from build123d import *

# Parameters (mm, degrees)
BOSS_EXTRUDE1_DEPTH = 10
FILLET1_R           = 5
CUT_EXTRUDE1_REACH  = 273.931
SKETCH2_R           = 1.5
SKETCH3_R           = 3
CUT_EXTRUDE2_DEPTH  = 2


with BuildPart() as part:
    # Sketch1 → Boss-Extrude1 (new body)
    with BuildSketch(Plane.XY):
        with BuildLine():
            Line((20, 35.715152736), (170, 35.715152736))
            ThreePointArc((170, 35.715152736), (184.142135624, 29.85728836), (190, 15.715152736))
            Line((190, 15.715152736), (190, -189.284847264))
            ThreePointArc((190, -189.284847264), (188.535533906, -192.82038117), (185, -194.284847264))
            Line((185, -194.284847264), (5, -194.284847264))
            ThreePointArc((5, -194.284847264), (1.464466094, -192.82038117), (0, -189.284847264))
            Line((0, -189.284847264), (0, 15.715152736))
            ThreePointArc((0, 15.715152736), (5.857864376, 29.85728836), (20, 35.715152736))
        make_face()
    extrude(amount=BOSS_EXTRUDE1_DEPTH)

    # Fillet1
    fillet1_edges = [part.edges().sort_by_distance(p)[0] for p in [
        (1.464466094, -192.82038117, 10),
        (95, -194.284847264, 10),
        (188.535533906, -192.82038117, 10),
        (190, -86.784847264, 10),
        (184.142135624, 29.85728836, 10),
        (95, 35.715152736, 10),
        (5.857864376, 29.85728836, 10),
        (0, -86.784847264, 10),
    ]]
    fillet(fillet1_edges, radius=FILLET1_R)

    # Sketch2 → Cut-Extrude1 (cut, up to next)
    with BuildSketch(Plane.XY.offset(10), mode=Mode.PRIVATE) as cut_extrude1_sk1:
        with Locations((20, -174.284847264)):
            Circle(SKETCH2_R)
    cut_extrude1_tool1 = extrude(cut_extrude1_sk1.sketch, amount=-CUT_EXTRUDE1_REACH, mode=Mode.PRIVATE) & part.part
    # Sketch2 → Cut-Extrude1 (cut, up to next)
    with BuildSketch(Plane.XY.offset(10), mode=Mode.PRIVATE) as cut_extrude1_sk2:
        with Locations((170, -174.284847264)):
            Circle(SKETCH2_R)
    cut_extrude1_tool2 = extrude(cut_extrude1_sk2.sketch, amount=-CUT_EXTRUDE1_REACH, mode=Mode.PRIVATE) & part.part
    # Sketch2 → Cut-Extrude1 (cut, up to next)
    with BuildSketch(Plane.XY.offset(10), mode=Mode.PRIVATE) as cut_extrude1_sk3:
        with Locations((170, 15.715152736)):
            Circle(SKETCH2_R)
    cut_extrude1_tool3 = extrude(cut_extrude1_sk3.sketch, amount=-CUT_EXTRUDE1_REACH, mode=Mode.PRIVATE) & part.part
    # Sketch2 → Cut-Extrude1 (cut, up to next)
    with BuildSketch(Plane.XY.offset(10), mode=Mode.PRIVATE) as cut_extrude1_sk4:
        with Locations((20, 15.715152736)):
            Circle(SKETCH2_R)
    cut_extrude1_tool4 = extrude(cut_extrude1_sk4.sketch, amount=-CUT_EXTRUDE1_REACH, mode=Mode.PRIVATE) & part.part
    add(cut_extrude1_tool1.solids().sort_by_distance((20, -174.284847, 10))[0], mode=Mode.SUBTRACT)
    add(cut_extrude1_tool2.solids().sort_by_distance((170, -174.284847, 10))[0], mode=Mode.SUBTRACT)
    add(cut_extrude1_tool3.solids().sort_by_distance((170, 15.715153, 10))[0], mode=Mode.SUBTRACT)
    add(cut_extrude1_tool4.solids().sort_by_distance((20, 15.715153, 10))[0], mode=Mode.SUBTRACT)

    # Sketch3 → Cut-Extrude2 (cut)
    with BuildSketch(Plane.XY.offset(10)):
        with Locations((20, 15.715152736)):
            Circle(SKETCH3_R)
        with Locations((170, 15.715152736)):
            Circle(SKETCH3_R)
        with Locations((170, -174.284847264)):
            Circle(SKETCH3_R)
        with Locations((20, -174.284847264)):
            Circle(SKETCH3_R)
    extrude(amount=-CUT_EXTRUDE2_DEPTH, mode=Mode.SUBTRACT)


solid = part.part
Part model, mm, in its own coordinate system. A direction names the side the tool comes from. Coordinates: 2 decimals unless noted, no trailing zeros.
(1) Pin check, flat tips, straight feed: pin 1 Ø1.5 at (x, z) = (107.5, 6) entering from -Y; pin 2 Ø3 at (x, y) = (170, 16.5) entering from +Z; pin 3 Ø4 at (x, z) = (71, 8.5) entering from -Y. Stop position of each tip, or through.
Check sheet entries:
pin 1: stops at y = -194.28
pin 2: stops at z = 8
pin 3: stops at y = -194.05
(2) Pull direction X, two halves, no side cores. Call faces 1 (the face through (96, -78, 10)), 2 (the face through (1, -85, 8)), 3 (the face through (21, 14, 8)): pulls with the +X half, pulls with the -X half, needs draft (parallel to the pull), parting line crosses it, or undercut.
Check sheet entries:
face 1: needs draft
face 2: pulls with the -X half
face 3: undercut
(3) Tool access for faces 4 (the face through (94, 35.715, 2)), 5 (the face through (17.62, -176.11, 9.01)): list every direction of +Z, -Z, +X, -X, +Y, -Y with a clear straight run to the whole face (end or side of a thin tool).
Check sheet entries:
face 4: +Z, -Z, +X, -X, +Y
face 5: +Z
(4) Probe L1, parallel to Y at x = 20, z = 1.5; L2, parallel to Y at x = 20, z = 6; L3, parallel to X at y = -67.5, z = 8. List the from-to ranges inside material, lowest first.
Check sheet entries:
L1: y = -194.28 to -175.78, -172.78 to 14.22, 17.22 to 35.72
L2: y = -194.18 to -175.78, -172.78 to 14.22, 17.22 to 35.61
L3: x = 1 to 189
